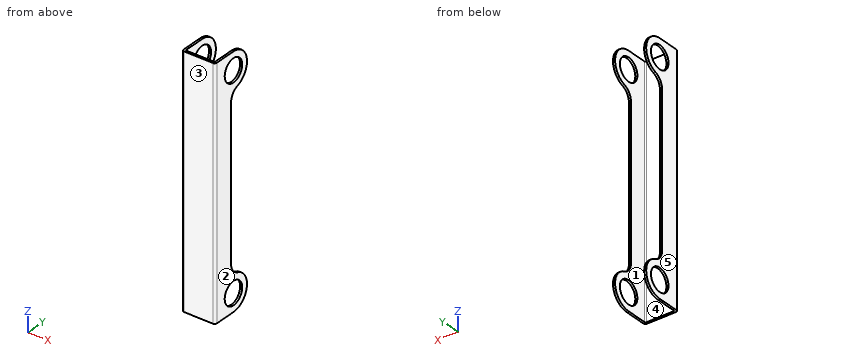
Autodesk Inventor part; units mm, degrees
ref_plane "Arbeitsebene1" through (40, 5, 292.5) normal (0, 0, 1) x (1, 0, 0)
ref_plane "Arbeitsebene2" through (0, 0, 0) normal (1, 0, 0) x (0, 1, 0)
ref_plane "XZ Plane" through (0, 0, 0) normal (0, 1, 0) x (-1, 0, 0)
sketch "Skizze1" plane through (0, 0, 0) normal (0, 0, 1) x (1, 0, 0)
  line L0 (0, 60) -> (0, -10)
  line L1 (-56, 0) -> (56, 0)
  line L2 (-56, 0) -> (56, 0)
  line L3 (0, -10) -> (0, 60)
  line L4 (-40, 0) -> (40, 0)
  line L5 (-40, 0) -> (-40, 50)
  line L6 (40, 0) -> (40, 50)
  line L7 (-35, 50) -> (-35, 5)
  line L8 (-35, 5) -> (35, 5)
  line L9 (35, 5) -> (35, 50)
  line L10 (-40, 50) -> (-35, 50)
  line L11 (40, 50) -> (35, 50)
  point P0 (0, 0)
  point P1 (0, 0)
  dimension "d0" = 80
  dimension "d1" = 50
  dimension "d2" = 50
  dimension "d4" = 5
extrude "Extrusion1" add sketch "Skizze1" along normal blind 585
fillet "Rundung1" radius 2.5 2 edges at (-35, 5, 292.5) (35, 5, 292.5)
fillet "Rundung1" radius 5 2 edges at (40, 0, 292.5) (-40, 0, 292.5)
sketch "Skizze2" plane through (40, 50, 585) normal (1, 0, 0) x (0, 0, -1)
  line L0 (585, -45) -> (0, -45)
  line L1 (585, -45) -> (585, 0)
  line L2 (585, 0) -> (0, 0)
  line L3 (0, -45) -> (0, 0)
  line L4 (0, -45) -> (0, -50)
  line L5 (0, -50) -> (585, -50)
  line L6 (585, -50) -> (585, -45)
  line L7 (585, -45) -> (0, -45)
  arc A0 (85, 7.5) -> (0, 7.5) centre (42.5, 7.5) ccw
  line L8 (0, 7.5) -> (0, 0)
  line L9 (85, 7.5) -> (85, 0)
  point P0 (585, -50)
  dimension "d9" = 85
  dimension "d10" = 100
  dimension "d11" = 42.5
extrude "Extrusion2" add sketch "Skizze2" against normal blind 5 contours L8 A0 L9 L2
sketch "Skizze3" plane through (40, 5, 0) normal (1, 0, 0) x (0, 0, -1)
  line L0 (0, 0) -> (-585, 0)
  line L1 (0, 0) -> (0, 45)
  line L2 (0, 45) -> (-500, 45)
  line L3 (-500, 45) -> (-500, 52.5)
  arc A0 (-500, 52.5) -> (-585, 52.5) centre (-542.5, 52.5) ccw
  line L4 (-585, 0) -> (-585, 52.5)
  circle A1 centre (-542.5, 52.5) radius 27.5
  point P0 (0, -5)
  dimension "d14" = 55
extrude "Extrusion3" cut sketch "Skizze3" against normal blind 5 contours A1
ref_plane "Arbeitsebene1" through (40, 5, 292.5) normal (0, 0, 1) x (1, 0, 0)
ref_plane "Arbeitsebene2" through (0, 0, 0) normal (1, 0, 0) x (0, 1, 0)
mirror "Spiegeln1" about plane through (40, 5, 292.5) normal (0, 0, 1) of "Extrusion2", "Extrusion3"
mirror "Spiegeln2" about plane through (0, 0, 0) normal (1, 0, 0) of "Extrusion2", "Extrusion3", "Spiegeln1"
fillet "Rundung2" radius 30 4 edges at (37.5, 50, 500) (-37.5, 50, 500) (-37.5, 50, 85) (37.5, 50, 85)
properties part number "Randschiene 2L"
Part model, mm, in its own coordinate system. Face numbers are marked on the shaded views. A direction names the side the tool comes from. Round coordinates to 2 decimals unless told otherwise and drop trailing zeros. Write each loop counter-clockwise with the first axis right and the second up, starting at its lowest first coordinate (ties: lowest second). Pieces come first, ordered by that corner, then holes. Notation, with made-up numbers: (48.25, 39.5) -> (52.25, 39.5) arc R19 cw to (52.25, 52.5) -> close; hole circle Ø5 at (-11, 72). An arc over 180 degrees is marked (long way). Return JSON: item names as keys, results as strings. Group by question number.
Q1. Saw through at A-A on z = 42.5. Write the cut outline in (x, y), plus the area to 3 significant figures.
Q2. Pin check, flat tips, straight feed: pin 1 (8 mm diameter, centred on x = -27.5, z = 139.5, fed in from -Y); pin 2 (4 mm diameter, centred on x = 38, z = 341, fed in from +Y); pin 3 (12 mm diameter, centred on x = 7, z = 258, fed in from +Y). Stop position of each tip, or through.
Q3. Saw through at D-D on z = 250.5. Write the cut outline in (x, y).
Q4. Which spindle directions (+Z, -Z, +X, -X, +Y, -Y) get a long thin tool onto all of the face, cutting with end or side? Do the marked faces 1 and 2. Say none if no direction does.
Q5. Mould opens along X. For the marked faces 3, 4 and 5 say: pulls with the +X half, pulls with the -X half, needs draft (parallel to the pull), parting line crosses it, or undercut.
Q6. Saw through at B-B on y = 13.5. Write the cut outline in (x, z), plus the area to 3 significant figures.
Q7. Probe L1, parallel to X at y = 18, z = 117.5; L2, parallel to Z at x = 38, y = 57; L3, parallel to Y at x = -20, z = 200. List the from-to ranges inside material, lowest first. Write a range as [from, to].
Q8. Saw through at C-C on y = 78. State how many separate pieces and enclosed holes the cut face has, plus the area to 3 significant figures.
Answer:
{
 "1": {"outline": "(-40, 5) arc R5 ccw to (-35, 0) -> (35, 0) arc R5 ccw to (40, 5) -> (40, 30) -> (35, 30) -> (35, 7.5) arc R2.5 cw to (32.5, 5) -> (-32.5, 5) arc R2.5 cw to (-35, 7.5) -> (-35, 30) -> (-40, 30) -> close; (-40, 85) -> (-35, 85) -> (-35, 100) -> (-40, 100) -> close; (35, 85) -> (40, 85) -> (40, 100) -> (35, 100) -> close", "area": "792 mm2"},
 "2": {"pin 1": "y = 0", "pin 2": "y = 50", "pin 3": "y = 5"},
 "3": {"outline": "(-40, 5) arc R5 ccw to (-35, 0) -> (35, 0) arc R5 ccw to (40, 5) -> (40, 50) -> (35, 50) -> (35, 7.5) arc R2.5 cw to (32.5, 5) -> (-32.5, 5) arc R2.5 cw to (-35, 7.5) -> (-35, 50) -> (-40, 50) -> close"},
 "4": {"face 1": "+Z, -Z, +Y", "face 2": "+Z, -Z, +X, +Y, -Y"},
 "5": {"face 3": "needs draft", "face 4": "undercut", "face 5": "pulls with the -X half"},
 "6": {"outline": "(-40, 0) -> (-35, 0) -> (-35, 585) -> (-40, 585) -> close; (35, 0) -> (40, 0) -> (40, 585) -> (35, 585) -> close", "area": "5,850 mm2"},
 "7": {"L1": "[-40, -35], [35, 40]", "L2": "[0, 15], [70, 92.16], [492.84, 515], [570, 585]", "L3": "[0, 5]"},
 "8": {"separate pieces": "8", "enclosed holes": "0", "area": "756 mm2"}
}
